The model under review builds one solid part; all positions refer to its coordinate system, in mm. A direction names the side the tool comes from. Coordinates: 2 decimals unless noted, no trailing zeros. Write each loop counter-clockwise with the first axis right and the second up, starting at its lowest first coordinate (ties: lowest second). Pieces come first, ordered by that corner, then holes. Notation, with made-up numbers: (63.25, 82) -> (76.25, 82) arc R21 ccw to (76.25, 121) -> close; hole circle Ø6 at (16.5, 62). An arc over 180 degrees is marked (long way). Write each question's results on one line, items separated by ' | '.
```python
from build123d import *

# Parameters (mm, degrees)
SKETCH1_W           = 78
SKETCH1_H           = 58
BOSS_EXTRUDE1_DEPTH = 19
SKETCH2_R           = 4.75
CUT_EXTRUDE1_DEPTH  = 5
CUT_EXTRUDE2_START  = -5
SKETCH2_3_R         = 2.75
CUT_EXTRUDE2_DEPTH  = 95.040395799


with BuildPart() as part:
    # Sketch1 → Boss-Extrude1 (new body)
    with BuildSketch(Plane.XY):
        with Locations((39, 29)):
            Rectangle(SKETCH1_W, SKETCH1_H)
    extrude(amount=BOSS_EXTRUDE1_DEPTH)

    # Sketch2 → Cut-Extrude1 (cut)
    with BuildSketch(Plane.XY.offset(19)):
        with Locations((39, 44)):
            Circle(SKETCH2_R)
    extrude(amount=-CUT_EXTRUDE1_DEPTH, mode=Mode.SUBTRACT)

    # Sketch2<3> → Cut-Extrude2 (cut, through all)
    with BuildSketch(Plane.XY.offset(19).offset(CUT_EXTRUDE2_START)):
        with Locations((39, 44)):
            Circle(SKETCH2_3_R)
    extrude(amount=-CUT_EXTRUDE2_DEPTH, mode=Mode.SUBTRACT)


solid = part.part
```
Q1. Add section B-B (y = 44). Write out the cut boundary in (x, z), plus the area to 3 significant figures.
Solution:
outline: (0, 0) -> (36.25, 0) -> (36.25, 14) -> (34.25, 14) -> (34.25, 19) -> (0, 19) -> close; (41.75, 0) -> (78, 0) -> (78, 19) -> (43.75, 19) -> (43.75, 14) -> (41.75, 14) -> close | area: 1,360 mm²
Q2. Add section C-C (z = 17.5). Write out the cut boundary in (x, y), plus the area to 3 significant figures.
Solution:
outline: (0, 0) -> (78, 0) -> (78, 58) -> (0, 58) -> close; hole circle Ø9.5 at (39, 44) | area: 4,450 mm²
Q3. For line 1 (Y direction, x = 39, z = 15.05); line 2 (Y direction, x = 39, z = 9), list the stretches that pass through material, from the lowest coordinate up. Write a range as from..to.
Solution:
line 1: 0..39.25, 48.75..58 | line 2: 0..41.25, 46.75..58
Q4. Add section A-A (x = 39). Write out the cut boundary in (y, z), plus the area to 4 significant figures.
Solution:
outline: (0, 0) -> (41.25, 0) -> (41.25, 14) -> (39.25, 14) -> (39.25, 19) -> (0, 19) -> close; (46.75, 0) -> (58, 0) -> (58, 19) -> (48.75, 19) -> (48.75, 14) -> (46.75, 14) -> close | area: 977.5 mm²
Q5. Machinability: for faces 1 (the cylindrical face through (41.554, 48.005, 16.535)), 2 (the flat face through (0, 29, 9)), which of the approach directions +Z, -Z, +X, -X, +Y, -Y give a long, thin tool a straight path to every point of the face, cutting with its end or side? Answer none if there is none.
Solution:
face 1: +Z | face 2: +Z, -Z, -X, +Y, -Y
Q6. Draft analysis for pull direction X (two halves, no side actions). For faces 3 (the flat face through (39, 41, 14)), 4 (the flat face through (78, 29, 9)), 5 (the flat face through (38, 0, 9)), state which applies: pulls with the +X half, pulls with the -X half, needs draft (parallel to the pull), parting line crosses it, or undercut.
Solution:
face 3: undercut | face 4: pulls with the +X half | face 5: needs draft
